Work out the finished part from the listing and answer in its coordinate system (mm). A direction names the side the tool comes from. Round coordinates to 2 decimals unless told otherwise and drop trailing zeros. Write each loop counter-clockwise with the first axis right and the second up, starting at its lowest first coordinate (ties: lowest second). Pieces come first, ordered by that corner, then holes. Notation, with made-up numbers: M 28.25,17.25 L 34.25,17.25 A27 ccw 34.25,53.25 Z; hole C 88.25,59.25 d10. An arc over 180 degrees is marked long. Answer in a Markdown table with one row per item.
```python
from build123d import *

# Parameters (mm, degrees)
SKETCH_1_W               = 56
SKETCH_1_H               = 34.4
EXTRUDE_1_DEPTH          = 2
SKETCH_2_W               = 8
SKETCH_2_H               = 2
EXTRUDE_2_DEPTH          = 6
MIRROR_2_COPY_1_SKETCH_W = 8
MIRROR_2_COPY_1_SKETCH_H = 2
MIRROR_2_COPY_1_DEPTH    = 6
EXTRUDE_3_DEPTH          = 8
EXTRUDE_4_DEPTH          = 8
EXTRUDE_5_DEPTH          = 8
CUT_EXTRUDE_1_DEPTH      = 10
SKETCH_8_W               = 69.954255789
SKETCH_8_H               = 15.282314342
SKETCH_8_W_2             = 75.120108524
SKETCH_8_H_2             = 7.103047511
CUT_EXTRUDE_3_DEPTH      = 2
CUT_EXTRUDE_3_DEPTH_BACK = 3


with BuildPart() as part:
    # 草图1 → 凸台-拉伸1 (new body)
    with BuildSketch(Plane.XY):
        Rectangle(SKETCH_1_W, SKETCH_1_H)
    extrude(amount=EXTRUDE_1_DEPTH)

    # 草图2 → 凸台-拉伸2 (add)
    with BuildSketch(Plane.XZ.offset(17.2)):
        with Locations((-18, 1)):
            Rectangle(SKETCH_2_W, SKETCH_2_H)
    extrude_2 = extrude(amount=EXTRUDE_2_DEPTH)

    # 镜向1: 凸台-拉伸2 across plane
    add(extrude_2.mirror(Plane.ZX))

    # 镜向2: 凸台-拉伸2 across plane
    add(extrude_2.mirror(Plane(origin=(0, 0, 0), x_dir=(0, 0, 1), z_dir=(1, 0, 0))))

    # 镜向2 copy 1 sketch → 镜向2 copy 1 (add)
    with BuildSketch(Plane(origin=(0, 17.2, 0), x_dir=(-1, 0, 0), z_dir=(0, 1, 0))):
        with Locations((-18, 1)):
            Rectangle(MIRROR_2_COPY_1_SKETCH_W, MIRROR_2_COPY_1_SKETCH_H)
    extrude(amount=MIRROR_2_COPY_1_DEPTH)

    # 草图4 → 凸台-拉伸3 (add)
    with BuildSketch(Plane(origin=(-14, 0, 0), x_dir=(0, 0, -1), z_dir=(1, 0, 0))):
        Polygon((-2, -23.2), (-2, -21.7), (-3, -21.7), align=None)
    extrude(amount=-EXTRUDE_3_DEPTH)

    # 草图5 → 凸台-拉伸4 (add)
    with BuildSketch(Plane(origin=(22, 0, 0), x_dir=(0, 0, -1), z_dir=(1, 0, 0))):
        Polygon((-2, -21.7), (-3, -21.7), (-2, -23.2), align=None)
        Polygon((-2, 23.2), (-2, 21.7), (-3, 21.7), align=None)
    extrude(amount=-EXTRUDE_4_DEPTH)

    # 草图6 → 凸台-拉伸5 (add)
    with BuildSketch(Plane(origin=(-14, 0, 0), x_dir=(0, 0, -1), z_dir=(1, 0, 0))):
        Polygon((-2, 23.2), (-2, 21.7), (-3, 21.7), align=None)
    extrude(amount=-EXTRUDE_5_DEPTH)

    # 草图7 → 切除-拉伸1 (cut)
    with BuildSketch(Plane.XY.offset(2)):
        with BuildLine():
            Line((-9.5, -8), (-9.5, 8))
            ThreePointArc((-9.5, 8), (-8, 9.5), (-6.5, 8))
            Line((-6.5, 8), (-6.5, -8))
            ThreePointArc((-6.5, -8), (-8, -9.5), (-9.5, -8))
        make_face()
        with BuildLine():
            Line((-21.5, -8), (-21.5, 8))
            ThreePointArc((-21.5, 8), (-20, 9.5), (-18.5, 8))
            Line((-18.5, 8), (-18.5, -8))
            ThreePointArc((-18.5, -8), (-20, -9.5), (-21.5, -8))
        make_face()
        with BuildLine():
            Line((6.5, -8), (6.5, 8))
            ThreePointArc((6.5, 8), (8, 9.5), (9.5, 8))
            Line((9.5, 8), (9.5, -8))
            ThreePointArc((9.5, -8), (8, -9.5), (6.5, -8))
        make_face()
        with BuildLine():
            Line((21.5, -8), (21.5, 8))
            ThreePointArc((21.5, 8), (20, 9.5), (18.5, 8))
            Line((18.5, 8), (18.5, -8))
            ThreePointArc((18.5, -8), (20, -9.5), (21.5, -8))
        make_face()
    extrude(amount=-CUT_EXTRUDE_1_DEPTH, mode=Mode.SUBTRACT)

    # 草图8 → 切除-拉伸3 (cut, two sides)
    with BuildSketch(Plane.XY.offset(2)) as cut_extrude_3_sk:
        with Locations((4.63474967, 27.841157171)):
            Rectangle(SKETCH_8_W, SKETCH_8_H)
        with Locations((-0.3158592, -23.751523756)):
            Rectangle(SKETCH_8_W_2, SKETCH_8_H_2)
    extrude(amount=CUT_EXTRUDE_3_DEPTH, mode=Mode.SUBTRACT)
    extrude(cut_extrude_3_sk.sketch, amount=-CUT_EXTRUDE_3_DEPTH_BACK, mode=Mode.SUBTRACT)


solid = part.part
```
1. The part is cut by section D-D (x = -20). Determine the outline of the cut face in (y, z), plus the area to 3 significant figures.
Calculated:
| item | result |
|---|---|
| outline | M -20.2,0 L -9.5,0 L -9.5,2 L -20.2,2 Z; M 9.5,0 L 20.2,0 L 20.2,2 L 9.5,2 Z |
| area | 42.8 mm² |
2. Consider line 1 along X through (y, z) = (0, 1.45); line 2 along X through (y, z) = (-9, 0.25); line 3 along Y through (x, z) = (-21, 1.5). Determine where each line is inside the solid, lowest interval first. Write a range as from..to.
Calculated:
| item | result |
|---|---|
| line 1 | x = -28..-21.5, -18.5..-9.5, -6.5..6.5, 9.5..18.5, 21.5..28 |
| line 2 | x = -28..-21.12, -18.88..-9.12, -6.88..6.88, 9.12..18.88, 21.12..28 |
| line 3 | y = -20.2..-9.12, 9.12..20.2 |
3. Determine the mould class of faces 4 (the flat face through (22, -19, 1)), 5 (the flat face through (9.5, 0, 1)), 6 (the flat face through (-25, -17.2, 1)) for opening direction X: released by +X, released by -X, zero draft, split by the parting line, or undercut.
Calculated:
| item | result |
|---|---|
| face 4 | released by +X |
| face 5 | undercut |
| face 6 | zero draft |
4. A tool of negligible diameter and unlimited length cuts with its end or side. For faces 1 (the flat face through (-22, 19, 1)), 2 (the flat face through (25, 17.2, 1)), 3 (the flat face through (-21.5, 0, 1)), from which of +Z, -Z, +X, -X, +Y, -Y can it reach the whole face along a straight path? Write none if from no direction.
Calculated:
| item | result |
|---|---|
| face 1 | +Z, -Z, -X, +Y |
| face 2 | +Z, -Z, +X, +Y |
| face 3 | +Z, -Z |
5. The part is cut by section C-C (z = 1.3). Count the separate pieces of the cut face and the enclosed holes in it, plus the area to 3 significant figures.
Calculated:
| item | result |
|---|---|
| separate pieces | 1 |
| enclosed holes | 4 |
| area | 1,800 mm² |
6. The part is cut by section A-A (x = 8). Determine the outline of the cut face in (y, z).
Calculated:
| item | result |
|---|---|
| outline | M -17.2,0 L -9.5,0 L -9.5,2 L -17.2,2 Z; M 9.5,0 L 17.2,0 L 17.2,2 L 9.5,2 Z |
7. Given pin 1 (1 mm diameter, centred on x = 25, z = 1, fed in from -Y); pin 2 (1 mm diameter, centred on x = -24, z = 1, fed in from +Y); pin 3 (0.6 mm diameter, centred on y = 18, z = 1, fed in from -X), each flat-ended and moving along its own axis, determine where each tip first touches the part or whether it passes through.
Calculated:
| item | result |
|---|---|
| pin 1 | stops at y = -17.2 |
| pin 2 | stops at y = 17.2 |
| pin 3 | stops at x = -22 |
8. The part is cut by section B-B (y = 3). Determine the outline of the cut face in (x, z).
Calculated:
| item | result |
|---|---|
| outline | M -28,0 L -21.5,0 L -21.5,2 L -28,2 Z; M -18.5,0 L -9.5,0 L -9.5,2 L -18.5,2 Z; M -6.5,0 L 6.5,0 L 6.5,2 L -6.5,2 Z; M 9.5,0 L 18.5,0 L 18.5,2 L 9.5,2 Z; M 21.5,0 L 28,0 L 28,2 L 21.5,2 Z |
